Geometry: see drawing. Coordinates: mm, zero at the bounding-box minimum. A direction names the side the tool comes from. Round coordinates to 2 decimals unless told otherwise and drop trailing zeros. Loops run counter-clockwise (first coordinate to the right, second up) from the corner with the lowest first, then second, coordinate; pieces in that order, holes last.
(1) Cut plane A-A, the plane y = 49. Output: boundary loops of the cut face in (x, z).
(2) Access query for the marked faces 1, 2 and 3. Directions: +Z, -Z, +X, -X, +Y, -Y. A direction counts if a zero-diameter tool reaches every point of the face in a straight line with its end or side. Return the directions, or none.
(3) Line query: line 1 (Y direction, x = 28, z = 107.9); line 2 (Z direction, x = 5.5, y = 23.5); line 3 (X direction, y = 7, z = 108.35). Output: solid intervals per line, ascending.
(4) Cut plane D-D, the plane y = 37. Output: boundary loops of the cut face in (x, z), and give its area (3 significant figures).
(5) First-contact query: pin 1 Ø5 at (y, z) = (34, 49.5) entering from +X; pin 2 Ø2.5 at (x, y) = (7, 28) entering from -Z; pin 3 Ø1.5 at (x, y) = (35, 8) entering from -Z; pin 4 Ø4.5 at (x, y) = (49, 28) entering from +Z. Flat tips, straight axial feed; report the tip coordinate or a pass-through.
(6) Cut plane C-C, the plane z = 43.5. Output: boundary loops of the cut face in (x, y).
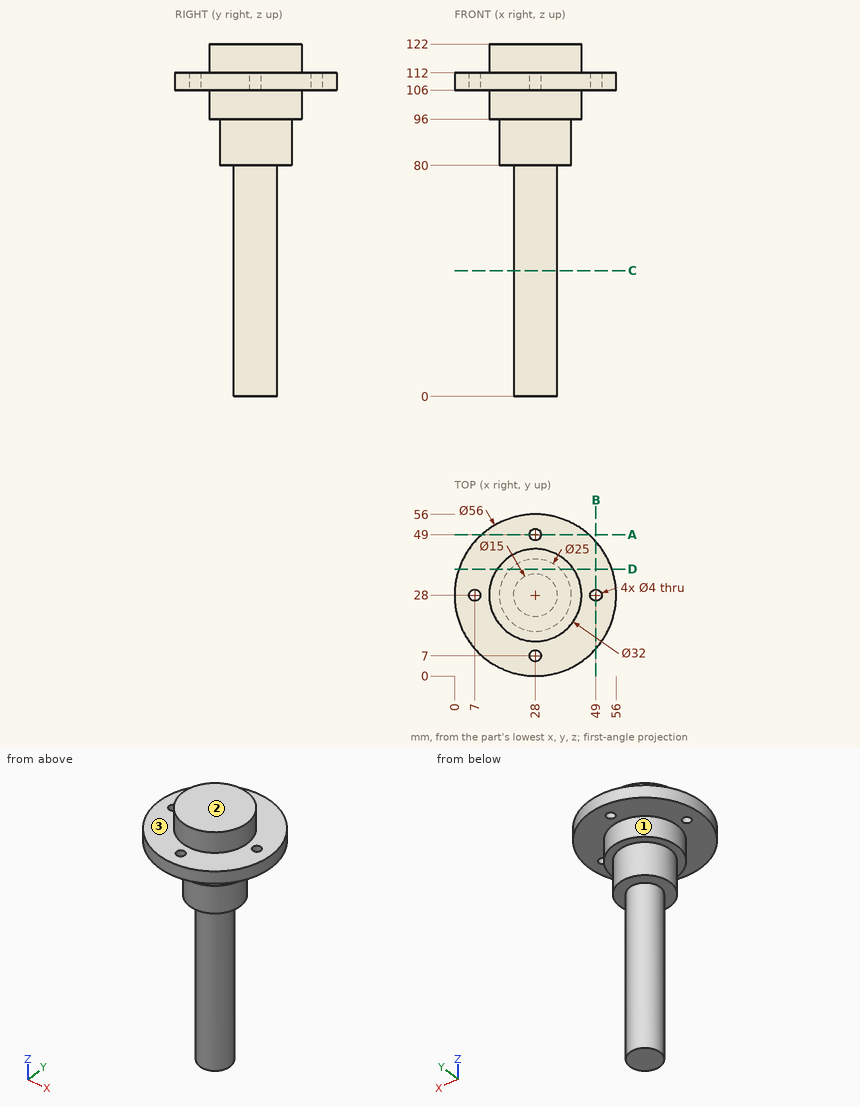
Reported:
1. outline: (9.48, 106) - (26, 106) - (26, 112) - (9.48, 112) - close; (30, 106) - (46.52, 106) - (46.52, 112) - (30, 112) - close
2. face 1: -Z
2. face 2: +Z, +X, -X, +Y, -Y
2. face 3: +Z
3. line 1: y = 0 to 5, 9 to 47, 51 to 56
3. line 2: z = 106 to 112
3. line 3: x = 9.48 to 26, 30 to 46.52
4. outline: (1.49, 106) - (14.77, 106) - (14.77, 96) - (19.33, 96) - (19.33, 80) - (36.67, 80) - (36.67, 96) - (41.23, 96) - (41.23, 106) - (54.51, 106) - (54.51, 112) - (41.23, 112) - (41.23, 122) - (14.77, 122) - (14.77, 112) - (1.49, 112) - close
4. area: 1,120 mm2
5. pin 1: stops at x = 34.63
5. pin 2: passes through
5. pin 3: stops at z = 106
5. pin 4: stops at z = 112
6. outline: circle Ø15 at (28, 28)
